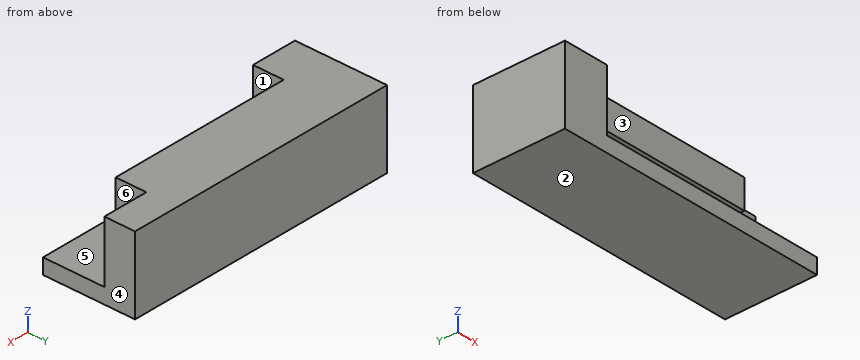
```python
from build123d import *

# Parameters (mm, degrees)
SKETCH2_W           = 18
SKETCH2_H           = 5
BOSS_EXTRUDE1_DEPTH = 6
CUT_EXTRUDE1_DEPTH  = 15
CUT_EXTRUDE2_REACH  = 13.916
SKETCH4_W           = 3
SKETCH4_H           = 2


with BuildPart() as part:
    # Sketch2 → Boss-Extrude1 (new body)
    with BuildSketch(Plane(origin=(0, 0, 0), x_dir=(1, 0, 0), z_dir=(0, 1, 0))):
        Rectangle(SKETCH2_W, SKETCH2_H)
    extrude(amount=BOSS_EXTRUDE1_DEPTH)

    # Sketch3 → Cut-Extrude1 (cut)
    with BuildSketch(Plane(origin=(9, 0, 0), x_dir=(0, 0, -1), z_dir=(1, 0, 0))):
        Polygon((-2.5, 0), (1.5, 0), (1.5, 4), (-0.6, 4), (-0.6, 2), (-2.5, 2), align=None)
    extrude(amount=-CUT_EXTRUDE1_DEPTH, mode=Mode.SUBTRACT)

    # Sketch4 → Cut-Extrude2 (cut, up to next)
    with BuildSketch(Plane.XY.offset(2.5), mode=Mode.PRIVATE) as cut_extrude2_sk1:
        with Locations((7.5, 3)):
            Rectangle(SKETCH4_W, SKETCH4_H)
    cut_extrude2_tool1 = extrude(cut_extrude2_sk1.sketch, amount=-CUT_EXTRUDE2_REACH, mode=Mode.PRIVATE) & part.part
    add(cut_extrude2_tool1.solids().sort_by_distance((7.5, 3, 2.5))[0], mode=Mode.SUBTRACT)


solid = part.part
```
Check sheet for the modelled part. Datum: model origin and axes. Units: mm. Face numbers are marked on the shaded views. A direction names the side the tool comes from. Coordinates: 2 decimals unless noted, no trailing zeros. Order: outer loops, then holes, each group sorted by start corner. A loop starts at its lowest first (then second) coordinate and runs counter-clockwise, first axis right, second up. Notation, with made-up numbers: M 76.5,-33.75 L 124.5,-33.75 A18 cw 124.5,-28.75 Z; hole C 72,39.5 d5. An arc over 180 degrees is marked long. Write each question's results on one line, items separated by ' | '. Start each with the question number.
1. Go/stop test with flat-tipped pins: P1, Ø1, axis at x = 2, z = 2, coming from the -Y side; P2, Ø1.5, axis at y = 3, z = 1, coming from the +X side. Record where each tip stops, or that it passes through.
2. Mould release check, pull along Z, two halves, no side actions. Record for the marked faces 1, 2 and 3: +Z half, -Z half, draft (parallel to the pull), parting line (faces both ways), or undercut.
3. Cross-section at A-A on x = 2. Record the cut outline in (y, z).
4. Access from +Z, -Z, +X, -X, +Y, -Y to the whole of each face (thin tool, end or side, straight path). Record for the marked faces 4, 5 and 6.
5. Cross-section at D-D on z = 0. Record the cut outline in (x, y).
6. Cross-section at C-C on y = 1.5. Record the cut outline in (x, z), and give its area (3 significant figures).
7. Cross-section at B-B on z = 1.75. Record the cut outline in (x, y).
8. Material ranges on probe 1 along Z at (x, y) = (-4.5, 3.9); probe 2 along Y at (x, z) = (-2, 2.15); probe 3 along Y at (x, z) = (3.5, -0.45), recorded low to high.
Checks:
1) P1: stops at y = 2 | P2: stops at x = 6
2) face 1: undercut | face 2: -Z half | face 3: draft
3) outline: M 0,-2.5 L 6,-2.5 L 6,2.5 L 2,2.5 L 2,0.6 L 4,0.6 L 4,-1.5 L 0,-1.5 Z
4) face 4: +Z, -Z, +X, +Y, -Y | face 5: +X, -Y | face 6: +Z, +X, -Y
5) outline: M -9,0 L -6,0 L -6,4 L 9,4 L 9,6 L -9,6 Z
6) outline: M -9,-2.5 L 9,-2.5 L 9,-1.5 L -6,-1.5 L -6,2.5 L -9,2.5 Z | area: 30.0 mm²
7) outline: M -9,0 L -6,0 L -6,2 L 6,2 L 6,4 L 9,4 L 9,6 L -9,6 Z
8) probe 1: z = -2.5 to -1.5, 0.6 to 2.5 | probe 2: y = 2 to 6 | probe 3: y = 4 to 6
